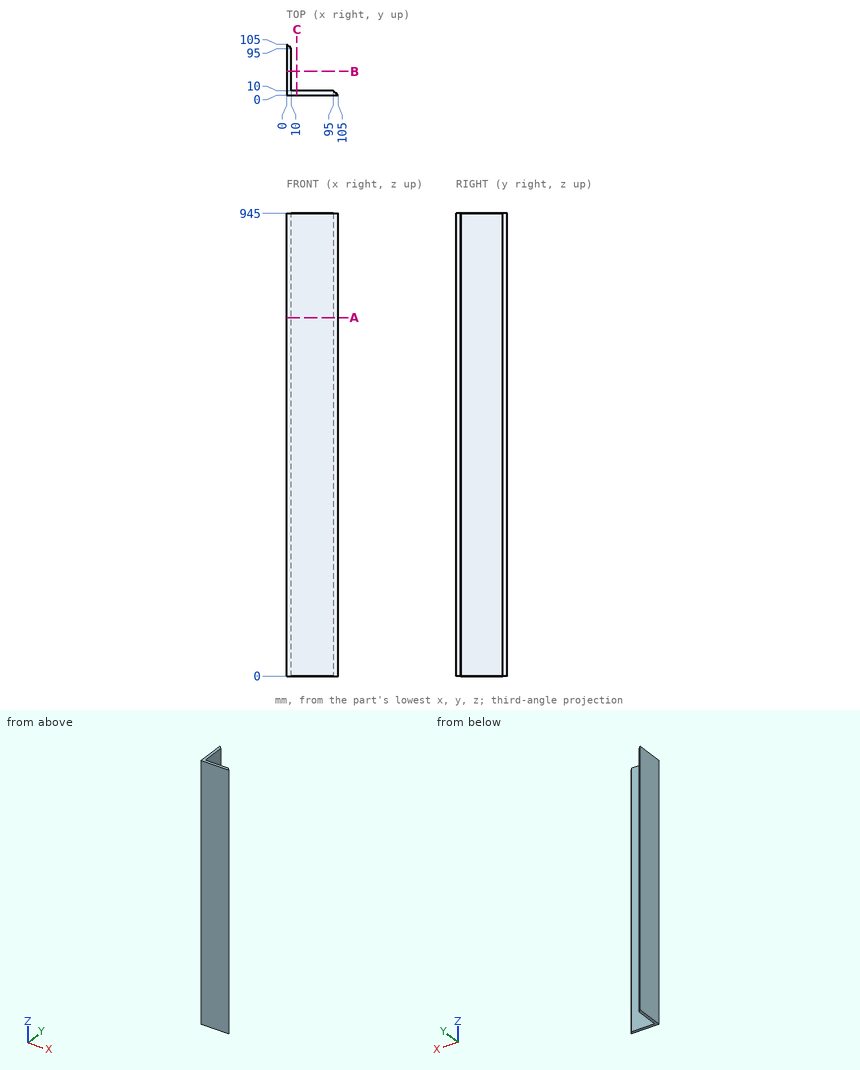
Could you check a few things on this drawing? It's one solid part, dimensions in mm from its lowest x, y, z. Give positions to 0.01 mm unless a question says otherwise; leave off trailing zeros. Order: outer loops, then holes, each group sorted by start corner. A loop starts at its lowest first (then second) coordinate and runs counter-clockwise, first axis right, second up. Notation, with made-up numbers: (76.25, 40.25) -> (134.25, 40.25) arc R12 ccw to (134.25, 51.25) -> close; hole circle Ø9 at (36, 16.25). An arc over 180 degrees is marked (long way). Answer in a Markdown table with one row per item. Add a question column.
Item 1: Please list where these lines run through material, in increasing order: probe 1 along X at (y, z) = (15.5, 248); probe 2 along Y at (x, z) = (7.5, 399).
Item 2: Imagine slicing it at B-B (y = 49). List the corners of the cut face in (x, z) for me, and give its area (3 significant figures).
Item 3: I'm going to push flat-ended pins straight in: P1, Ø5, axis at y = 18, z = 294.5, coming from the +X side; P2, Ø10, axis at x = 50, z = 526, coming from the +Y side. Where does each tip first touch, or does it pass through?
Item 4: Imagine slicing it at A-A (z = 732). List the corners of the cut face in (x, y) for me, and give its area (3 significant figures).
Result:
| question | item | result |
|---|---|---|
| 1 | probe 1 | 0 to 10 |
| 1 | probe 2 | 0 to 97.5 |
| 2 | outline | (0, 0) -> (10, 0) -> (10, 945) -> (0, 945) -> close |
| 2 | area | 9,450 mm2 |
| 3 | P1 | x = 10 |
| 3 | P2 | y = 10 |
| 4 | outline | (0, 0) -> (105, 0) -> (95, 10) -> (10, 10) -> (10, 95) -> (0, 105) -> close |
| 4 | area | 1,900 mm2 |
